Could you check a few things on this model? Use its own coordinates, in mm. A direction names the side the tool comes from. Round coordinates to 2 decimals unless told otherwise and drop trailing zeros. Write each loop counter-clockwise with the first axis right and the second up, starting at its lowest first coordinate (ties: lowest second). Pieces come first, ordered by that corner, then holes.
Autodesk Inventor part; units mm, degrees
ref_plane "YZ Plane" through (0, 0, 0) normal (1, 0, 0) x (0, 1, 0)
ref_plane "XZ Plane" through (0, 0, 0) normal (0, 1, 0) x (-1, 0, 0)
ref_plane "XY Plane" through (0, 0, 0) normal (0, 0, 1) x (1, 0, 0)
ref_plane "Work Plane3" through (68.5837, 137.6229, 5) normal (0, 0, -1) x (0.999249, -0.038749, 0)
sketch "Sketch3" plane through (68.5837, 137.6229, 5) normal (0, 0, -1) x (0.999249, -0.038749, 0)
  line L0 (-44.3, -40.7514) -> (-37.8, -40.7514)
  line L1 (-37.8, -8.3514) -> (-37.8, -40.7514)
  line L2 (-44.3, -8.3514) -> (-37.8, -8.3514)
  line L3 (-44.3, -8.3514) -> (-44.3, -40.7514)
  circle A0 centre (-41.4, -14.5514) radius 1.75 construction
  circle A1 centre (-41.4, -34.5514) radius 1.75 construction
  line L4 (-25, -40.7514) -> (-18.5, -40.7514)
  line L5 (-18.5, -8.3514) -> (-18.5, -40.7514)
  line L6 (-25, -8.3514) -> (-18.5, -8.3514)
  line L7 (-25, -8.3514) -> (-25, -40.7514)
  circle A2 centre (-21.4, -14.5514) radius 1.75 construction
  circle A3 centre (-21.4, -34.5514) radius 1.75 construction
  line L8 (-18.5, -40.7514) -> (-45.9422, -40.7514)
  line L9 (-45.9422, -40.7514) -> (-45.9422, -6.7531)
  line L10 (-45.9422, -6.7531) -> (-18.5, -6.7531)
  line L11 (-18.5, -6.7531) -> (-18.5, -40.7514)
  circle A4 centre (-41.4, -14.5514) radius 1.75
  circle A5 centre (-41.4, -34.5514) radius 1.45
  circle A6 centre (-41.4, -14.5514) radius 1.45
  circle A7 centre (-21.4, -14.5514) radius 1.45
  circle A8 centre (-21.4, -34.5514) radius 1.45
  line L12 (-17.9, -8.3514) -> (-17.9, -40.7514)
  line L13 (-18.5, -40.7514) -> (-11.5, -40.7514)
  line L14 (-11.5, -40.7514) -> (-11.5, -8.3514)
  line L15 (-11.5, -8.3514) -> (-18.5, -8.3514)
  line L16 (-18.5, -8.3514) -> (-18.5, -40.7514)
  point P0 (-63.1994, 140.177)
  dimension "d12" = 2.9
  dimension "d13" = 2.9
  dimension "d14" = 2.9
  dimension "d15" = 2.9
  dimension "d16" = 7
extrude "Extrusion3" add sketch "Sketch3" along normal blind 4 contours L3 L2 L1 L0 | L8 L9 L10 L11 L6 L7 L1 L2 L3 | L7 L6 L5 L4 | L5 L15 L12 L13 | L12 L15 L14 L13 | A4
ref_plane "Work Plane4" through (22.9376, 146.1511, 1) normal (-0.038749, -0.999249, 0) x (0.999249, -0.038749, 0)
sketch "Sketch4" plane through (22.9376, 146.1511, 1) normal (-0.038749, -0.999249, 0) x (0.999249, -0.038749, 0)
  line L0 (27.4422, 4) -> (0, 4)
  line L1 (0, 4) -> (0, 0)
  line L2 (27.4422, 0) -> (0, 0)
  arc A0 (20.387, 12.6266) -> (19.8094, 12.1273) centre (20.8422, 11.5162) ccw construction
  arc A1 (19.616, 12.0055) -> (19.8094, 12.1273) centre (19.5942, 12.2545) ccw construction
  line L3 (19.616, 12.0055) -> (19.2704, 11.9753) construction
  arc A2 (19.2704, 11.9753) -> (19.0422, 11.7262) centre (19.2922, 11.7262) ccw construction
  line L4 (19.0422, 11.7262) -> (19.0422, 11.2738) construction
  arc A3 (19.0422, 11.2738) -> (19.2704, 11.0247) centre (19.2922, 11.2738) ccw construction
  line L5 (19.2704, 11.0247) -> (19.637, 10.9927) construction
  arc A4 (19.8267, 10.8768) -> (19.637, 10.9927) centre (19.6152, 10.7436) ccw construction
  arc A5 (19.8267, 10.8768) -> (20.387, 10.4059) centre (20.8422, 11.5162) ccw construction
  arc A6 (20.5422, 10.1746) -> (20.387, 10.4059) centre (20.2922, 10.1746) ccw construction
  line L6 (20.5422, 10.1746) -> (20.5422, 9.5) construction
  line L7 (20.5422, 9.5) -> (20.0422, 9) construction
  line L8 (20.0422, 9) -> (9.0422, 9) construction
  line L9 (9.0422, 9) -> (8.5422, 9.5) construction
  line L10 (8.5422, 9.5) -> (8.5422, 10.1746) construction
  arc A7 (8.6974, 10.4059) -> (8.5422, 10.1746) centre (8.7922, 10.1746) ccw construction
  arc A8 (8.6974, 10.4059) -> (9.2577, 10.8768) centre (8.2422, 11.5162) ccw construction
  arc A9 (9.4474, 10.9927) -> (9.2577, 10.8768) centre (9.4692, 10.7436) ccw construction
  line L11 (9.4474, 10.9927) -> (9.814, 11.0247) construction
  arc A10 (9.814, 11.0247) -> (10.0422, 11.2738) centre (9.7922, 11.2738) ccw construction
  line L12 (10.0422, 11.2738) -> (10.0422, 11.7262) construction
  arc A11 (10.0422, 11.7262) -> (9.814, 11.9753) centre (9.7922, 11.7262) ccw construction
  line L13 (9.814, 11.9753) -> (9.4684, 12.0055) construction
  arc A12 (9.275, 12.1273) -> (9.4684, 12.0055) centre (9.4902, 12.2545) ccw construction
  arc A13 (9.275, 12.1273) -> (8.6974, 12.6266) centre (8.2422, 11.5162) ccw construction
  arc A14 (8.5422, 12.8579) -> (8.6974, 12.6266) centre (8.7922, 12.8579) ccw construction
  line L14 (8.5422, 12.8579) -> (8.5422, 14) construction
  line L15 (8.5422, 14) -> (1.6422, 14) construction
  line L16 (1.6422, 14) -> (1.0422, 13.4) construction
  line L17 (1.0422, 13.4) -> (1.0422, 10) construction
  arc A15 (1.0422, 9.2) -> (1.0422, 10) centre (0.7422, 9.6) ccw construction
  line L18 (1.0422, 9.2) -> (1.0422, 4.6) construction
  line L19 (1.0422, 4.6) -> (1.6422, 4) construction
  line L20 (1.6422, 4) -> (8.1422, 4) construction
  line L21 (8.1422, 4) -> (8.5422, 4.4) construction
  line L22 (8.5422, 4.4) -> (20.5422, 4.4) construction
  line L23 (20.5422, 4.4) -> (20.9422, 4) construction
  line L24 (20.9422, 4) -> (27.4422, 4) construction
  line L25 (27.4422, 4) -> (28.0422, 4.6) construction
  line L26 (28.0422, 4.6) -> (28.0422, 13.4) construction
  line L27 (28.0422, 13.4) -> (27.4422, 14) construction
  line L28 (27.4422, 14) -> (20.5422, 14) construction
  line L29 (20.5422, 14) -> (20.5422, 12.8579) construction
  arc A16 (20.387, 12.6266) -> (20.5422, 12.8579) centre (20.2922, 12.8579) ccw construction
  line L30 (0, 4) -> (34.4422, 4)
  line L31 (34.4422, 4) -> (28.2422, 4)
  line L32 (28.2422, 4) -> (28.2422, 16.2)
  line L33 (28.2422, 16.2) -> (34.4422, 16.2)
  line L34 (34.4422, 16.2) -> (34.4422, 4)
  line L35 (28.2422, 16.2) -> (23.0467, 16.2)
  line L36 (23.0467, 16.2) -> (23.0467, 14.2)
  line L37 (23.0467, 14.2) -> (28.2422, 14.2)
  line L38 (28.2422, 14.2) -> (28.2422, 16.2)
  circle A17 centre (31.3422, 9) radius 2
  line L39 (27.4422, 4) -> (27.4422, 0)
  line L40 (27.4422, 0) -> (34.4422, 0)
  line L41 (34.4422, 0) -> (34.4422, 4)
  line L42 (34.4422, 4) -> (27.4422, 4)
  line L43 (27.4422, 4) -> (27.4422, 0)
  point P0 (-17.2572, -1)
  dimension "d17" = 0.2
  dimension "d18" = 0.2
  dimension "d19" = 2
  dimension "d20" = 4
extrude "Extrusion4" add sketch "Sketch4" against normal blind 5
ref_plane "Work Plane5" through (22.9376, 146.1511, 1) normal (-0.038749, -0.999249, 0) x (0.999249, -0.038749, 0)
sketch "Sketch6" plane through (22.9376, 146.1511, 1) normal (-0.038749, -0.999249, 0) x (0.999249, -0.038749, 0)
  line L0 (27.4422, 4) -> (0, 4)
  line L1 (0, 4) -> (0, 0)
  line L2 (27.4422, 0) -> (0, 0)
  line L3 (27.4422, 4) -> (27.4422, 0)
  line L4 (28.2422, 14.2) -> (23.0467, 14.2)
  line L5 (23.0467, 14.2) -> (28.2422, 14.2)
  line L6 (28.2422, 14.2) -> (28.2422, 4)
  line L7 (28.2422, 4) -> (23.0467, 4)
  line L8 (23.0467, 4) -> (23.0467, 14.2)
  line L9 (27.4422, 4) -> (28.2422, 4)
  line L10 (27.4422, 4) -> (27.4422, 0)
  line L11 (34.4422, 0) -> (27.4422, 0)
  line L12 (34.4422, 4) -> (34.4422, 0)
  line L13 (28.2422, 4) -> (34.4422, 4)
  circle A0 centre (31.3422, 9) radius 2
  line L14 (34.4422, 16.2) -> (23.0467, 16.2)
  line L15 (23.0467, 16.2) -> (23.0467, 14.2)
  line L16 (23.0467, 14.2) -> (28.2422, 14.2)
  line L17 (28.2422, 4) -> (28.2422, 14.2)
  line L18 (34.4422, 16.2) -> (34.4422, 0)
  line L19 (28.2422, 4) -> (0, 4)
  line L20 (0, 4) -> (0, 0)
  line L21 (0, 0) -> (34.4422, 0)
  point P0 (-17.2572, -1)
extrude "Extrusion6" add sketch "Sketch6" along normal blind 7 contours L3 L2 L1 L0 | L7 L13 L12 L11 L3 | L6 L4 L15 L14 L18 L13
ref_plane "Work Plane6" through (22.6664, 139.1564, 1) normal (-0.038749, -0.999249, 0) x (0.999249, -0.038749, 0)
sketch "Sketch7" plane through (22.6664, 139.1564, 1) normal (-0.038749, -0.999249, 0) x (0.999249, -0.038749, 0)
  circle A0 centre (31.3422, 9) radius 2
  line L0 (28.2422, 4) -> (0, 4)
  line L1 (0, 4) -> (0, 0)
  line L2 (0, 0) -> (34.4422, 0)
  line L3 (23.0467, 14.2) -> (23.0467, 16.2)
  line L4 (28.2422, 4) -> (34.4422, 4)
  line L5 (23.0467, 14.2) -> (28.2422, 14.2)
  line L6 (28.2422, 14.2) -> (28.2422, 4)
  line L7 (28.2422, 4) -> (23.0467, 4)
  line L8 (23.0467, 4) -> (23.0467, 14.2)
  line L9 (34.4422, 0) -> (34.4422, 16.2)
  line L10 (34.4422, 16.2) -> (23.0467, 16.2)
  line L11 (23.0467, 16.2) -> (23.0467, 14.2)
  line L12 (23.0467, 14.2) -> (28.2422, 14.2)
  line L13 (28.2422, 14.2) -> (28.2422, 4)
  point P0 (-17.2572, -1)
extrude "Extrusion7" add sketch "Sketch7" along normal blind 2
sketch "Sketch5" plane through (22.5889, 137.1579, 1) normal (0.038749, 0.999249, 0) x (0.999249, -0.038749, 0)
  circle A0 centre (31.3422, -9) radius 2
  line L0 (28.5922, -10.5877) -> (28.5922, -7.4123)
  line L1 (28.5922, -7.4123) -> (31.3422, -5.8246)
  line L2 (31.3422, -5.8246) -> (34.0922, -7.4123)
  line L3 (34.0922, -7.4123) -> (34.0922, -10.5877)
  line L4 (34.0922, -10.5877) -> (31.3422, -12.1754)
  line L5 (31.3422, -12.1754) -> (28.5922, -10.5877)
  point P0 (-17.2572, 1)
  point P1 (31.3422, -9)
  dimension "d23" = 0
  dimension "d24" = 5.5
extrude "Extrusion5" cut sketch "Sketch5" along normal blind 4
sketch "Sketch8" plane through (68.5837, 137.6229, 1) normal (0, 0, -1) x (-0.999249, 0.038749, 0)
  line L0 (22.8955, 11.7531) -> (11.5, 11.7531)
  line L1 (12.6, 1.7531) -> (16.6, 1.7531)
  circle A0 centre (14.6, 14.0688) radius 1.45
  point P0 (63.1994, -140.177)
  dimension "d31" = 2.9
extrude "Extrusion8" cut sketch "Sketch8" against normal up to surface
sketch "Sketch9" plane through (22.5889, 137.1579, 1) normal (-0.038749, -0.999249, 0) x (0.999249, -0.038749, 0)
  circle A0 centre (15.7007, 11.4189) radius 1.45
  point P0 (-17.2572, -1)
extrude "Extrusion9" cut sketch "Sketch9" against normal blind 5
equation "\"d32\" = d31"
properties part number "30_cellSTORM_translation_y"
Q1. I'm going to push flat-ended pins straight in: pin 1 Ø3 at (x, z) = (36.5, 5.5) entering from +Y; pin 2 Ø4 at (x, y) = (48.54, 172.98) entering from +Z; pin 3 Ø1.5 at (x, z) = (31.5, 4) entering from +Y. Where does each tip first touch, or does it pass through?
Q2. Imagine slicing it at A-A, the plane z = 10.5. Write out the boundary of the cut face in (x, y), then the cut area to 3 significant figures.
Q3. If I drill on L1, parallel to Z at x = 47, y = 147; L2, parallel to Z at x = 49.5, y = 166; L3, parallel to X at y = 139.5, z = 12.5, over which ranges is the centre line in solid material (lowest first)?
Q4. On a 3-axis mill with a long thin cutter (end or side, diameter ignored), from which of +Z, -Z, +X, -X, +Y, -Y can I reach the whole of each face in a straight line? I mean faces 5 (the cylindrical face through (49.163, 153.374, 3.028)), 6 (the flat face through (51.236, 138.021, 10.022)), 7 (the flat face through (53.04, 149.988, 12.541)). Say none if no direction works.
Q5. Imagine slicing it at B-B, the plane z = 7.5. Write out the boundary of the cut face in (x, y), then the cut area to 3 significant figures.
Q6. Imagine slicing it at D-D, the plane y = 165.5. Write out the boundary of the cut face in (x, z).
Q7. Imagine slicing it at C-C, the plane x = 38.5. Write out the boundary of the cut face in (y, z).
Q8. We'd pull the mould along Z, two halves only. Please class faces 1 (the cylindrical face through (29.871, 173.146, 3.028)), 2 (the flat face through (51, 143, 17.2)), 3 (the flat face through (56.732, 137.808, 9.978)), 4 (the flat face through (51.117, 143.974, 10.029)): pulls with the +Z half, pulls with the -Z half, needs draft (parallel to the pull), parting line crosses it, or undercut.
Results found:
1. pin 1: stops at y = 179.7
1. pin 2: stops at z = 5
1. pin 3: stops at y = 179.87
2. outline: (45.62, 136.26) - (51.16, 136.05) - (51.31, 140.05) - (52.13, 140.02) - (52.51, 150.01) - (51.35, 150.05) - (50.89, 138.06) - (45.7, 138.26) - close; (56, 139.87) - (56.81, 139.84) - (56.66, 135.84) - (57.01, 135.82) - (57.55, 149.81) - (56.39, 149.86) - close
2. area: 36.5 mm2
3. L1: z = 1 to 5, 15.2 to 17.2
3. L2: z = 1 to 5
3. L3: x = 50.94 to 52.87, 55.22 to 57.15
4. face 5: +Z, -Z
4. face 6: -Y
4. face 7: +Z, +X, +Y
5. outline: (45.62, 136.26) - (52.74, 135.99) - (52.89, 139.99) - (55.23, 139.9) - (55.08, 135.9) - (57.01, 135.82) - (57.55, 149.81) - (51.35, 150.05) - (50.89, 138.06) - (45.7, 138.26) - close
5. area: 87.8 mm2
6. outline: (23.69, 1) - (58.16, 1) - (58.16, 5) - (23.69, 5) - close
7. outline: (136.54, 1) - (179.57, 1) - (179.57, 5) - (136.54, 5) - close
8. face 1: needs draft
8. face 2: pulls with the +Z half
8. face 3: undercut
8. face 4: undercut
